Source: CAD feature listing. Evaluate the final solid. Frame: model axes, mm. Face numbers are marked on the shaded views. A direction names the side the tool comes from. Coordinates: 2 decimals unless noted, no trailing zeros. Loops run counter-clockwise (first coordinate to the right, second up) from the corner with the lowest first, then second, coordinate; pieces in that order, holes last.
from build123d import *

# Parameters (mm, degrees)
SKETCH_1_W          = 135
SKETCH_1_H          = 87
EXTRUDE_1_DEPTH     = 37.8
SKETCH_2_W          = 135
SKETCH_2_H          = 87
SKETCH_2_W_2        = 126
SKETCH_2_H_2        = 78
EXTRUDE_2_DEPTH     = 43
CUT_EXTRUDE_1_DEPTH = 177.430978006
CUT_EXTRUDE_2_DEPTH = 4.5
CUT_EXTRUDE_3_DEPTH = 4.5
EXTRUDE_3_DEPTH     = 4.5
EXTRUDE_4_DEPTH     = 4
EXTRUDE_5_DEPTH     = 4


with BuildPart() as part:
    # 草图1 → 凸台-拉伸1 (new body)
    with BuildSketch(Plane(origin=(0, 0, 0), x_dir=(1, 0, 0), z_dir=(0, 1, 0))):
        with Locations((63, -34.5)):
            Rectangle(SKETCH_1_W, SKETCH_1_H)
        Polygon((0, 0), (4.5, 0), (4.5, 4.5), (61, 4.5), (61, -73.5), (4.5, -73.5), (4.5, -69), (0, -69), align=None, mode=Mode.SUBTRACT)
        Polygon((121.5, 4.5), (121.5, 0), (126, 0), (126, -69), (121.5, -69), (121.5, -73.5), (65, -73.5), (65, 4.5), align=None, mode=Mode.SUBTRACT)
    extrude(amount=EXTRUDE_1_DEPTH)

    # 草图2 → 凸台-拉伸2 (add)
    with BuildSketch(Plane(origin=(0, 37.8, 0), x_dir=(1, 0, 0), z_dir=(0, 1, 0))):
        with Locations((63, -34.5)):
            Rectangle(SKETCH_2_W, SKETCH_2_H)
        with Locations((63, -34.5)):
            Rectangle(SKETCH_2_W_2, SKETCH_2_H_2, mode=Mode.SUBTRACT)
    extrude(amount=EXTRUDE_2_DEPTH)

    # 草图3 → 切除-拉伸1 (cut, through all)
    with BuildSketch(Plane.XY.offset(78)):
        with BuildLine():
            Line((-4.5, 80.8), (130.5, 80.8))
            ThreePointArc((130.5, 80.8), (63, 43.9), (-4.5, 80.8))
        make_face()
    extrude(amount=-CUT_EXTRUDE_1_DEPTH, mode=Mode.SUBTRACT)

    # 草图4 → 切除-拉伸2 (cut)
    with BuildSketch(Plane.XY.offset(78)):
        with BuildLine():
            Line((53.65, 27.169085989), (46.585, 45.598112395))
            Line((46.585, 45.598112395), (79.415, 45.598112395))
            Line((79.415, 45.598112395), (72.35, 27.169085989))
            ThreePointArc((72.35, 27.169085989), (63, 20.74), (53.65, 27.169085989))
        make_face()
    extrude(amount=-CUT_EXTRUDE_2_DEPTH, mode=Mode.SUBTRACT)

    # 草图5 → 切除-拉伸3 (cut)
    with BuildSketch(Plane(origin=(65, 0, 0), x_dir=(0, 0, -1), z_dir=(1, 0, 0))):
        with BuildLine():
            Line((-73.5, 37.8), (-48.24, 37.8))
            Line((-48.24, 37.8), (-60.563675282, 26.103423436))
            ThreePointArc((-60.563675282, 26.103423436), (-66.535963079, 22.279815799), (-73.5, 20.94176249))
            Line((-73.5, 20.94176249), (-73.5, 37.8))
        make_face()
    extrude(amount=-CUT_EXTRUDE_3_DEPTH, mode=Mode.SUBTRACT)

    # 草图6 → 凸台-拉伸3 (add)
    with BuildSketch(Plane(origin=(0, 0, -9), x_dir=(-1, 0, 0), z_dir=(0, 0, -1))):
        with BuildLine():
            Line((-65.25, 0), (-60.75, 0))
            Line((-60.75, 0), (-60.75, 43.931572736))
            ThreePointArc((-60.75, 43.931572736), (-63, 43.9), (-65.25, 43.931572736))
            Line((-65.25, 43.931572736), (-65.25, 0))
        make_face()
    extrude(amount=EXTRUDE_3_DEPTH)

    # 草图7 → 凸台-拉伸4 (add)
    with BuildSketch(Plane.ZY.offset(4.5)):
        with BuildLine():
            Line((-9, 0), (12.15, 0))
            ThreePointArc((12.15, 0), (-2.805308422, 6.194691578), (-9, 21.15))
            Line((-9, 21.15), (-9, 0))
        make_face()
        with BuildLine():
            Line((78, 0), (78, 21.15))
            Line((78, 21.15), (43.3, 21.15))
            ThreePointArc((43.3, 21.15), (37.105308422, 6.194691578), (22.15, 0))
            Line((22.15, 0), (78, 0))
        make_face()
    extrude(amount=EXTRUDE_4_DEPTH)

    # 草图8 → 凸台-拉伸5 (add)
    with BuildSketch(Plane(origin=(0, 0, 0), x_dir=(0, 0, -1), z_dir=(1, 0, 0))):
        with BuildLine():
            Line((0, 6.347973112), (0, 0))
            Line((0, 0), (-31.3, 0))
            Line((-31.3, 0), (-69, 0))
            Line((-69, 0), (-69, 21.15))
            Line((-69, 21.15), (-31.3, 21.15))
            ThreePointArc((-31.3, 21.15), (-20.336879747, 3.83822655), (0, 6.347973112))
        make_face()
    extrude(amount=EXTRUDE_5_DEPTH)


solid = part.part
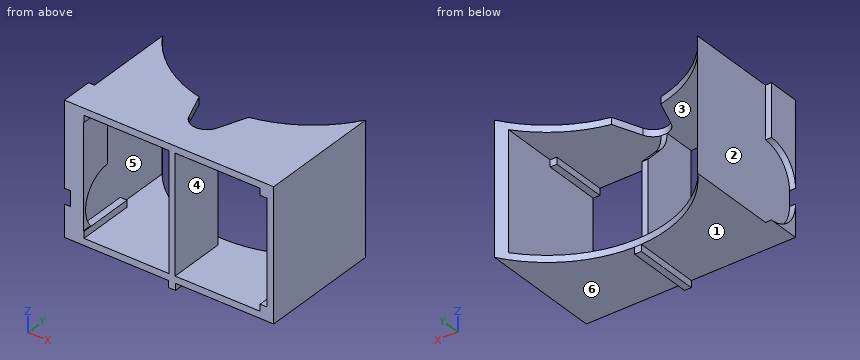
Q1. Contact query for flat-ended pins moving along their axis: pin 1 Ø5 at (x, z) = (1.5, 72) entering from +Y; pin 2 Ø2 at (y, z) = (13, -10.5) entering from -X; pin 3 Ø6 at (x, y) = (36.5, 8.5) entering from -Z. Output: stop coordinate, or through.
Q2. Section C-C, the plane x = 31. Return the cut outline in (y, z), plus the area to 3 significant figures.
Q3. Section B-B, the plane y = 68. Return the cut outline in (x, z).
Q4. Line query: line 1 along X through (y, z) = (25.5, 33.5); line 2 along X through (y, z) = (25.5, -2); line 3 along X through (y, z) = (48, 70). Output: solid intervals per line, ascending.
Q5. Section D-D, the plane y = 11. Count the separate pieces of the cut face and the enclosed holes in it, plus the area to 3 significant figures.
Q6. Section A-A, the plane z = 6. Return the cut outline in (x, y).
Q7. Draft query along X for the marked faces 1, 2 and 3. Return one class per face: +X half, -X half, draft (parallel to the pull), parting line (faces both ways), or undercut.
Q8. Access query for the marked faces 4, 5 and 6. Directions: +Z, -Z, +X, -X, +Y, -Y. A direction counts if a zero-diameter tool reaches every point of the face in a straight line with its end or side. Return the directions, or none.
Derived:
1. pin 1: stops at y = 75.78
1. pin 2: stops at x = 60.75
1. pin 3: stops at z = -9
2. outline: (0, -9) - (50.56, -9) - (50.56, -4.5) - (0, -4.5) - close; (0, 73.5) - (50.56, 73.5) - (50.56, 78) - (0, 78) - close
2. area: 455 mm2
3. outline: (-4.5, -9) - (5.69, -9) - (5.69, -4.5) - (0, -4.5) - (0, 73.5) - (5.69, 73.5) - (5.69, 78) - (-4.5, 78) - close; (120.31, -9) - (130.5, -9) - (130.5, 78) - (120.31, 78) - (120.31, 73.5) - (126, 73.5) - (126, -4.5) - (120.31, -4.5) - close
4. line 1: x = -4.5 to 0, 61 to 65, 126 to 130.5
4. line 2: x = -4.5 to 4.5, 61 to 65, 121.5 to 130.5
4. line 3: x = -4.5 to 0, 126 to 130.5
5. separate pieces: 1
5. enclosed holes: 2
5. area: 2,650 mm2
6. outline: (-8.5, 0) - (4, 0) - (4, 3.01) - (0, 3.01) - (0, 74.48) arc R80.19 cw to (-4.5, 80.8) - (-4.5, 0.91) - (-8.5, 0.91) - close; (61, 0) - (65, 0) - (65, 37.8) - (61, 37.8) - close; (126, 0) - (130.5, 0) - (130.5, 80.8) arc R80.19 cw to (126, 74.48) - close
7. face 1: draft
7. face 2: -X half
7. face 3: undercut
8. face 4: +Y, -Y
8. face 5: +Y
8. face 6: -Z, +X, +Y, -Y
